```python
from build123d import *

# Parameters (mm, degrees)
SKETCH_1_W          = 100
SKETCH_1_H          = 25
EXTRUDE_1_DEPTH     = 5
SKETCH_2_W          = 20
SKETCH_2_H          = 5
EXTRUDE_2_DEPTH     = 170
SKETCH_3_W          = 15
SKETCH_3_H          = 27.372730927
EXTRUDE_3_DEPTH     = 81
FILLET_1_R          = 5
SKETCH_6_W          = 15
SKETCH_6_H          = 23.851489588
FILLET_2_R          = 5
FILLET_3_R          = 5
SKETCH_5_W          = 4.727272728
SKETCH_5_H          = 4
CUT_EXTRUDE_3_DEPTH = 100


with BuildPart() as part:
    # 草图1 → 凸台-拉伸1 (new body)
    with BuildSketch(Plane.XY):
        Rectangle(SKETCH_1_W, SKETCH_1_H)
    extrude(amount=EXTRUDE_1_DEPTH)

    # 草图2 → 凸台-拉伸2 (add)
    with BuildSketch(Plane(origin=(0, 12.5, 0), x_dir=(1, 0, 0), z_dir=(0, 1, 0))):
        with Locations((0, -2.5)):
            Rectangle(SKETCH_2_W, SKETCH_2_H)
    extrude(amount=EXTRUDE_2_DEPTH)

    # 草图3 → 凸台-拉伸3 (add)
    with BuildSketch(Plane.XY.offset(5)):
        with Locations((0, 168.813634536)):
            Rectangle(SKETCH_3_W, SKETCH_3_H)
    extrude(amount=EXTRUDE_3_DEPTH)

    # 圆角1
    # the kernel refuses this fillet: 5 mm, written as the material it adds along each edge
    with BuildSketch(Plane(origin=(-7.5, 155.127269073, 5), x_dir=(-1, 0, 0), z_dir=(0, 1, 0)), Plane(origin=(7.5, 182.5, 5), x_dir=(1, 0, 0), z_dir=(0, -1, 0))) as fillet_1_piece_1:
        with BuildLine():
            CenterArc((5, 4.330127019), FILLET_1_R, 180, 60)
            Line((0, 4.330127019), (-0.1, 4.330127019))
            Line((-0.1, 4.330127019), (-0.1, 0))
            Line((-0.1, 0), (0, -0.1))
            ThreePointArc((0, -0.1), (1.25, -0.1), (2.45, -0.08660254))
            Line((2.45, -0.08660254), (2.5, 0))
        make_face()
    extrude(amount=27.372730927)

    # 扫描1: sweep along a path in 草图7
    with BuildLine(Plane(origin=(0, 0, 0), x_dir=(0, 0, -1), z_dir=(1, 0, 0))) as sweep_1_path:
        Line((-5, 24.875224673), (-67.976637777, 168.654354293))
    # 草图6 → 扫描1 (sweep)
    with BuildSketch(Plane.XY.offset(5)):
        with Locations((0, 24.875224673)):
            Rectangle(SKETCH_6_W, SKETCH_6_H)
    sweep(path=sweep_1_path.line)

    # 圆角2
    fillet_2_edges = [part.edges().sort_by_distance(p)[0] for p in [
        (-10, 12.5, 2.5),
        (10, 12.5, 2.5),
    ]]
    fillet(fillet_2_edges, radius=FILLET_2_R)

    # 圆角3
    fillet_3_edges = [part.edges().sort_by_distance(p)[0] for p in [
        (-50, 12.5, 2.5),
        (50, 12.5, 2.5),
        (50, -12.5, 2.5),
        (-50, -12.5, 2.5),
    ]]
    fillet(fillet_3_edges, radius=FILLET_3_R)

    # 草图5 → 切除-拉伸3 (cut)
    with BuildSketch(Plane(origin=(7.5, 0, 0), x_dir=(0, 0, -1), z_dir=(1, 0, 0))):
        with Locations((-67.976637777, 168.654354293)):
            Rectangle(SKETCH_5_W, SKETCH_5_H)
    extrude(amount=-CUT_EXTRUDE_3_DEPTH, mode=Mode.SUBTRACT)


solid = part.part
```
CAD build for the part. Positions are in the model's coordinates, mm. A direction names the side the tool comes from. Round coordinates to 2 decimals unless told otherwise and drop trailing zeros. Order: outer loops, then holes, each group sorted by start corner. A loop starts at its lowest first (then second) coordinate and runs counter-clockwise, first axis right, second up.
Q1. Slice it at C-C (z = 40.5). Write the cut outline in (x, y).
Q2. Slice it at A-A (x = 2.5). Write the cut outline in (y, z).
Q3. Slice it at D-D (y = 160.5). Write the cut outline in (x, z), and give its area (3 significant figures).
Q4. Wall check: L1, parallel to Y at x = 3, z = 68; L2, parallel to Z at x = 42, y = 7; L3, parallel to X at y = 174.5, z = 68. Give the ranges that are in metal, low to high.
Q5. Drop flat-ended pins along their axis: pin 1 (4 mm diameter, centred on y = 117.5, z = 1.5, fed in from +X); pin 2 (5.5 mm diameter, centred on x = 35, z = 3, fed in from +Y); pin 3 (24.5 mm diameter, centred on y = 135, z = 47.5, fed in from -X); pin 4 (2 mm diameter, centred on x = -3, y = 169.5, fed in from -Z). Give the stop position or say it passes through.
Q6. Slice it at B-B (y = 87). Write the cut outline in (x, z), and give its area (3 significant figures).
Q7. Two-plate mould, pull along Y, no slides. Class faces 1 (the cylindrical face through (48.57, 11, 2.54)), 2 (the flat face through (7.5, 135, 52)), 3 (the flat face through (0, 155.127, 31)): pulls with the +Y half, pulls with the -Y half, needs draft (parallel to the pull), parting line crosses it, or undercut.
Q8. Which spindle directions (+Z, -Z, +X, -X, +Y, -Y) get a long thin tool onto all of the face, cutting with end or side? Do faces 4 (the cylindrical face through (8.152, 169.005, 6.862)), 5 (the flat face through (0, 169, 70.34)), 6 (the flat face through (-30, 12.5, 2)). Say none if no direction does.
Results below:
1. outline: (-7.5, 94) - (7.5, 94) - (7.5, 117.85) - (-7.5, 117.85) - close; (-7.5, 155.13) - (7.5, 155.13) - (7.5, 182.5) - (-7.5, 182.5) - close
2. outline: (-12.5, 0) - (182.5, 0) - (182.5, 86) - (155.13, 86) - (155.13, 67.28) - (12.95, 5) - (-12.5, 5) - close; hole (36.8, 5) - (155.13, 5) - (155.13, 56.83) - close; hole (166.65, 65.61) - (170.65, 65.61) - (170.65, 70.34) - (166.65, 70.34) - close
3. outline: (-10, 0) - (10, 0) - (10, 5) arc R5 cw to (7.5, 9.33) - (7.5, 86) - (-7.5, 86) - (-7.5, 9.33) arc R5 cw to (-10, 5) - close
3. area: 1,320 mm2
4. L1: y = 155.13 to 166.65, 170.65 to 182.5
4. L2: z = 0 to 5
4. L3: x = -7.5 to 7.5
5. pin 1: stops at x = 10
5. pin 2: stops at y = 12.5
5. pin 3: stops at x = -7.5
5. pin 4: stops at z = 0
6. outline: (-10, 0) - (10, 0) - (10, 5) - (-10, 5) - close; (-7.5, 26.99) - (7.5, 26.99) - (7.5, 37.43) - (-7.5, 37.43) - close
6. area: 257 mm2
7. face 1: pulls with the +Y half
7. face 2: needs draft
7. face 3: undercut
8. face 4: +Z, +X, +Y, -Y
8. face 5: +X, -X
8. face 6: +Z, -Z, -X, +Y
